Answer from the drawing. Dimensions are ordinates in mm from the lowest x, y and z of the part. A direction names the side the tool comes from. Give positions to 0.01 mm unless a question says otherwise; leave off trailing zeros. Loops run counter-clockwise (first coordinate to the right, second up) from the corner with the lowest first, then second, coordinate; pieces in that order, holes last. Notation, with made-up numbers: (15, 87.25) - (36, 87.25) arc R11 cw to (36, 104.25) - close; hole circle Ø1 at (33.5, -4.75). An arc over 180 degrees is marked (long way). One line per question, with ' | ' between items. Start each with the question number.
1. Section A-A (z = 6.25) is taken. Determine the outline of the cut face in (x, y).
2. Find the intervals of material crossed by line 1 (X direction, y = 3.5, z = 7.5); line 2 (Z direction, x = 4.5, y = 2); line 3 (Z direction, x = 0.75, y = 4.5), in increasing order.
3. Each of these flat-tipped pins is pushed along its axis until it touches: pin 1 (2 mm diameter, centred on x = 1.5, y = 1, fed in from -Z); pin 2 (3 mm diameter, centred on y = 1, z = 3.5, fed in from -X); pin 3 (1 mm diameter, centred on x = 3.5, y = 3.5, fed in from +Z). Where does it stop, or does it pass through?
4. For a pull along Y with two mould halves and no side action, classify the marked faces 1, 2, 3 and 4 as released by +Y, released by -Y, zero draft, split by the parting line, or undercut.
5. Which of the six approach directions +Z, -Z, +X, -X, +Y, -Y give full straight-line access (tool end or side, diameter ignored) to the marked faces 5 and 6?
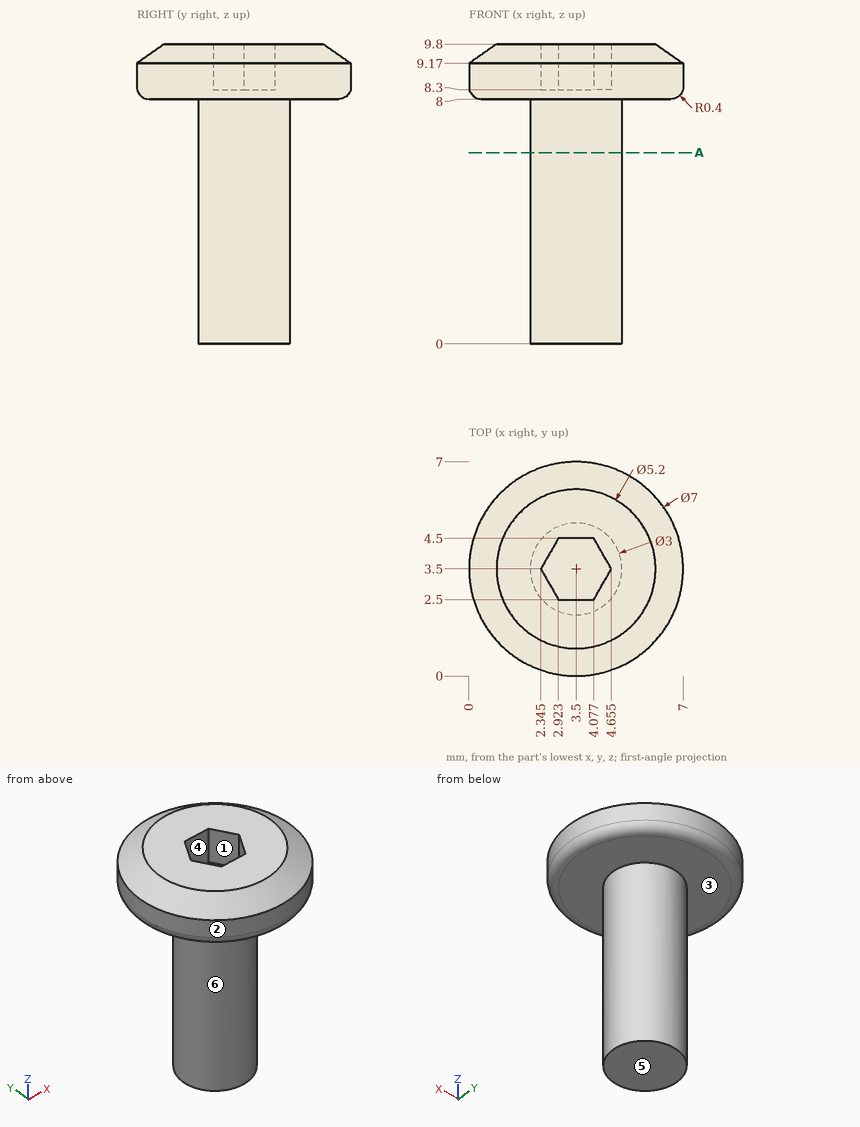
Conclusion:
1) outline: circle Ø3 at (3.5, 3.5)
2) line 1: 2 to 5 | line 2: 8 to 9.8 | line 3: 8 to 9.57
3) pin 1: z = 8 | pin 2: x = 2.38 | pin 3: z = 8.3
4) face 1: undercut | face 2: split by the parting line | face 3: zero draft | face 4: undercut
5) face 5: -Z, +X, -X, +Y, -Y | face 6: -Z
